```python
from build123d import *

# Parameters (mm, degrees)
CUT_EXTRUDE1_REACH          = 93.3
SKETCH8_R                   = 1.5875
TAP_DRILL_FOR_M3_TAP2_D     = 2.5
TAP_DRILL_FOR_M3_TAP2_DEPTH = 6
TAP_DRILL_FOR_M3_TAP2_TIP   = 0.751075774
TAP_DRILL_FOR_M4_TAP1_D     = 3.3
TAP_DRILL_FOR_M4_TAP1_DEPTH = 10
TAP_DRILL_FOR_M4_TAP1_TIP   = 0.991420021
CUT_EXTRUDE2_DEPTH          = 30
CIRPATTERN1_COUNT           = 2
CUT_EXTRUDE3_REACH          = 42.6
SKETCH19_R                  = 0.8


with BuildPart() as part:
    # Sketch3 → Revolve1 (revolve)
    with BuildSketch(Plane.XY):
        Polygon((208.579017697, -139.537446021), (250.685153788, -139.537446021), (259.278559985, -139.537446021), (259.278559985, -133.573704322), (238.427343436, -133.573704322), (221.978559985, -133.573704322), (221.978559985, -130.256968654), (197.978559985, -130.256968654), (197.978559985, -140.547506676), (167.978559985, -140.547506676), (167.978559985, -145.190124478), (205.151545348, -145.190124478), (205.151545348, -140.547506676), (208.579017697, -140.547506676), align=None)
    revolve(axis=Axis((227.370475166, -148.573704322, 0), (1, 0, 0)))

    # Sketch8 → Cut-Extrude1 (cut, up to next)
    with BuildSketch(Plane(origin=(259.278559985, 0, 0), x_dir=(0, 0, -1), z_dir=(1, 0, 0)), mode=Mode.PRIVATE) as cut_extrude1_sk1:
        with Locations((0, -136.573704322)):
            Circle(SKETCH8_R)
    cut_extrude1_tool1 = extrude(cut_extrude1_sk1.sketch, amount=-CUT_EXTRUDE1_REACH, mode=Mode.PRIVATE) & part.part
    add(cut_extrude1_tool1.solids().sort_by_distance((259.27856, -136.573704, 0))[0], mode=Mode.SUBTRACT)
    # Sketch8 → Cut-Extrude1 (cut, up to next)
    with BuildSketch(Plane(origin=(259.278559985, 0, 0), x_dir=(0, 0, -1), z_dir=(1, 0, 0)), mode=Mode.PRIVATE) as cut_extrude1_sk2:
        with Locations((0, -160.573704322)):
            Circle(SKETCH8_R)
    cut_extrude1_tool2 = extrude(cut_extrude1_sk2.sketch, amount=-CUT_EXTRUDE1_REACH, mode=Mode.PRIVATE) & part.part
    add(cut_extrude1_tool2.solids().sort_by_distance((259.27856, -160.573704, 0))[0], mode=Mode.SUBTRACT)

    # Tap Drill for M3 Tap2
    with Locations(Plane(origin=(259.278559985, 0, 0), x_dir=(0, 0, -1), z_dir=(1, 0, 0))):
        with Locations((-12, -148.573704322), (12, -148.573704322)):
            Hole(TAP_DRILL_FOR_M3_TAP2_D / 2, depth=TAP_DRILL_FOR_M3_TAP2_DEPTH)
            with Locations((0, 0, -(TAP_DRILL_FOR_M3_TAP2_DEPTH + TAP_DRILL_FOR_M3_TAP2_TIP / 2))):  # 118° drill point
                Cone(0, TAP_DRILL_FOR_M3_TAP2_D / 2, TAP_DRILL_FOR_M3_TAP2_TIP, mode=Mode.SUBTRACT)

    # Tap Drill for M4 Tap1
    with Locations(Plane.ZY.offset(-197.978559985)):
        with Locations((-12, -148.573704322), (12, -148.573704322)):
            Hole(TAP_DRILL_FOR_M4_TAP1_D / 2, depth=TAP_DRILL_FOR_M4_TAP1_DEPTH)
            with Locations((0, 0, -(TAP_DRILL_FOR_M4_TAP1_DEPTH + TAP_DRILL_FOR_M4_TAP1_TIP / 2))):  # 118° drill point
                Cone(0, TAP_DRILL_FOR_M4_TAP1_D / 2, TAP_DRILL_FOR_M4_TAP1_TIP, mode=Mode.SUBTRACT)

    # Sketch16 → Cut-Extrude2 (cut)
    with BuildSketch(Plane.ZY.offset(-197.978559985)):
        Polygon((-1.637133312, -127.583420636), (-21.615778458, -147.562065782), (-21.615778458, -136.774049127), align=None)
        Polygon((24.069809273, -155.63537923), (24.069809273, -147.131312047), (1.983531933, -169.217589388), align=None)
    extrude(amount=-CUT_EXTRUDE2_DEPTH, mode=Mode.SUBTRACT)

    # Sketch18 → Tap Drill for M5 Tap1 (revolve, cut)
    with BuildSketch(Plane(origin=(209.978559985, -137.259995823, -11.313708499), x_dir=(0, 0.707106781, 0.707106781), z_dir=(1, 0, 0))):
        Polygon((0, 0), (0, 5.2618073), (2.1, 4), (2.1, 0), align=None)
    tap_drill_for_m5_tap1 = revolve(axis=Axis((209.978559985, -132.769867763, -15.80383656), (0, -0.707106781, 0.707106781)), mode=Mode.SUBTRACT)

    # CirPattern1: Tap Drill for M5 Tap1 ×2 about axis
    cirpattern1_axis = Axis((205.151545348, -148.573704322, 0), (-1, 0, 0))
    for i in range(1, CIRPATTERN1_COUNT):
        add(tap_drill_for_m5_tap1.rotate(cirpattern1_axis, i * 360 / CIRPATTERN1_COUNT), mode=Mode.SUBTRACT)

    # Sketch19 → Cut-Extrude3 (cut, up to next)
    with BuildSketch(Plane(origin=(208.579017697, 0, 0), x_dir=(0, 0, -1), z_dir=(1, 0, 0)), mode=Mode.PRIVATE) as cut_extrude3_sk1:
        with Locations((5.586143571, -142.987560751)):
            Circle(SKETCH19_R)
    cut_extrude3_tool1 = extrude(cut_extrude3_sk1.sketch, amount=-CUT_EXTRUDE3_REACH, mode=Mode.PRIVATE) & part.part
    add(cut_extrude3_tool1.solids().sort_by_distance((208.579018, -142.987561, -5.586144))[0], mode=Mode.SUBTRACT)


solid = part.part
```
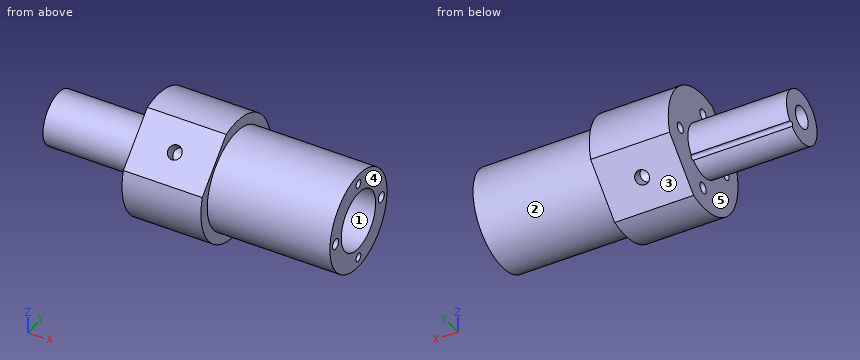
Source: CAD feature listing. Evaluate the final solid. Frame: model axes, mm. Face numbers are marked on the shaded views. A direction names the side the tool comes from. Coordinates: 2 decimals unless noted, no trailing zeros. Loops run counter-clockwise (first coordinate to the right, second up) from the corner with the lowest first, then second, coordinate; pieces in that order, holes last. Notation, with made-up numbers: M 30,70.25 L 41,70.25 A25 cw 41,88.25 Z; hole C 66.5,38 d6. An arc over 180 degrees is marked long. Use a Markdown table: item, result. Add a question column.
Q1. Draft query along Y for the marked faces 1, 2 and 3. Return one class per face: pulls with the +Y half, pulls with the -Y half, needs draft (parallel to the pull), parting line crosses it, or undercut.
Q2. First-contact query: pin 1 (8 mm diameter, centred on x = 183, z = 14, fed in from +Y); pin 2 (5 mm diameter, centred on y = -150, z = 3, fed in from +X); pin 3 (2 mm diameter, centred on y = -142.99, z = -5.59, fed in from +X); pin 4 (8 mm diameter, centred on x = 235.5, z = 10.5, fed in from +Y). Flat tips, straight axial feed; report the tip coordinate or a pass-through.
Q3. Section query B-B, the plane x = 176.5. Return loops of the section in (y, z), and give its area (3 significant figures).
Q4. Material intervals for L1, parallel to Z at x = 234.5, y = -149; L2, parallel to X at y = -149, z = -3.5; L3, parallel to Z at x = 189.5, y = -152.5, sorted ascending.
Q5. Section query A-A, the plane z = 0. State how many separate pieces and enclosed holes the cut face has, and give its area (3 significant figures).
Q6. Section query C-C, the plane z = 16. Return loops of the section in (x, y).
Q7. Access query for the marked faces 4 and 5. Directions: +Z, -Z, +X, -X, +Y, -Y. A direction counts if a zero-diameter tool reaches every point of the face in a straight line with its end or side. Return the directions, or none.
Result:
| question | item | result |
|---|---|---|
| 1 | face 1 | undercut |
| 1 | face 2 | parting line crosses it |
| 1 | face 3 | pulls with the +Y half |
| 2 | pin 1 | passes through |
| 2 | pin 2 | stops at x = 205.15 |
| 2 | pin 3 | stops at x = 208.58 |
| 2 | pin 4 | stops at y = -135.06 |
| 3 | outline | M -143.49,-6.21 A0.8 cw long -142.36,-5.09 A8.03 ccw long Z; hole C -148.57,0 d6.77 |
| 3 | area | 165 mm2 |
| 4 | L1 | z = -14.99 to -9.03, 9.03 to 14.99 |
| 4 | L2 | x = 167.98 to 205.15 |
| 4 | L3 | z = -7 to 7 |
| 5 | separate pieces | 4 |
| 5 | enclosed holes | 0 |
| 5 | area | 868 mm2 |
| 6 | outline | M 197.98,-155.2 L 221.98,-155.2 L 221.98,-139.66 L 197.98,-139.66 Z |
| 7 | face 4 | +Z, -Z, +X, +Y, -Y |
| 7 | face 5 | -X |
